Verification items for the finished model (mm, model axes). A direction names the side the tool comes from. Round coordinates to 2 decimals unless told otherwise and drop trailing zeros. Loops run counter-clockwise (first coordinate to the right, second up) from the corner with the lowest first, then second, coordinate; pieces in that order, holes last. Notation, with made-up numbers: (61, -27.75) -> (86, -27.75) arc R4 cw to (86, -21.75) -> close; hole circle Ø2 at (45.5, 15). An arc over 180 degrees is marked (long way). Use CSV: the item, a comma, the result in double quotes. Start each with the question number.
```python
from build123d import *

# Parameters (mm, degrees)
PAD_DEPTH = 35
FILLET_R  = 1


with BuildPart() as part:
    # Sketch → Pad (new body)
    with BuildSketch(Plane.XY):
        Polygon((0, 0), (0, 35), (-45.1, 35), (-45.1, 0), (-43.1, 0), (-43.1, 32), (-2, 32), (-2, 0), align=None)
    extrude(amount=PAD_DEPTH)

    # Fillet
    fillet_edges = [part.edges().sort_by_distance(p)[0] for p in [
        (0, 0, 17.5),
        (0, 35, 17.5),
        (0, 17.5, 0),
        (0, 17.5, 35),
        (-45.1, 35, 17.5),
        (-22.55, 35, 0),
        (-22.55, 35, 35),
        (-45.1, 0, 17.5),
        (-45.1, 17.5, 0),
        (-45.1, 17.5, 35),
    ]]
    fillet(fillet_edges, radius=FILLET_R)


solid = part.part
```
Q1. Depth check by flat-ended pin: pin 1 Ø12 at (x, z) = (-26.5, 26.5) entering from -Y. Enter the tip coordinate at first touch or a pass-through.
Q2. Thickness scan on L1, parallel to X at y = 6, z = 28; L2, parallel to Y at x = -35, z = 11.5. Record the ranges inside material, lowest first. Write a range as from..to.
Q3. Cross-section at C-C (x = -3). Record the boundary of the cut face in (y, z), and give its area (3 significant figures).
Q4. Cross-section at A-A (y = 6). Record the boundary of the cut face in (x, z), and give its area (3 significant figures).
Q5. Release check for a two-part mould opening along X. For faces 3 (the face through (-24.2, 32.2, 0)), 4 (the face through (0, 17, 17)), 5 (the face through (-2, 16, 17)) record: +X half, -X half, draft (parallel to the pull), parting line (faces both ways), or undercut.
Q6. Tool access check on faces 1 (the face through (-43.1, 16, 17)), 2 (the face through (-24.2, 32.2, 35)). Record the directions out of +Z, -Z, +X, -X, +Y, -Y that give a thin tool (end or side, any length) a straight path to the whole face; none if there is none.
Q7. Cross-section at B-B (z = 4.5). Record the boundary of the cut face in (x, y).
Answer list:
1,pin 1,"stops at y = 32"
2,L1,"x = -45.1..-43.1, -2..0"
2,L2,"y = 32..35"
3,outline,"(32, 0) -> (34, 0) arc R1 ccw to (35, 1) -> (35, 34) arc R1 ccw to (34, 35) -> (32, 35) -> close"
3,area,"105 mm2"
4,outline,"(-45.1, 1) arc R1 ccw to (-44.1, 0) -> (-43.1, 0) -> (-43.1, 35) -> (-44.1, 35) arc R1 ccw to (-45.1, 34) -> close; (-2, 0) -> (-1, 0) arc R1 ccw to (0, 1) -> (0, 34) arc R1 ccw to (-1, 35) -> (-2, 35) -> close"
4,area,"139 mm2"
5,face 3,"draft"
5,face 4,"+X half"
5,face 5,"undercut"
6,face 1,"+Z, -Z, -Y"
6,face 2,"+Z, +X, -X, +Y, -Y"
7,outline,"(-45.1, 1) arc R1 ccw to (-44.1, 0) -> (-43.1, 0) -> (-43.1, 32) -> (-2, 32) -> (-2, 0) -> (-1, 0) arc R1 ccw to (0, 1) -> (0, 34) arc R1 ccw to (-1, 35) -> (-44.1, 35) arc R1 ccw to (-45.1, 34) -> close"
